Build history of the part. All positions in model axes, mm. Coordinates: 2 decimals unless noted, no trailing zeros. Loops run counter-clockwise (first coordinate to the right, second up) from the corner with the lowest first, then second, coordinate; pieces in that order, holes last.
Item 1: Drill centre lines: line 1 along Y through (x, z) = (0.75, -1); line 2 along X through (y, z) = (-4.25, -1.5); line 3 along X through (y, z) = (-6.5, -0.5). Where is each one in solid material? Low to high.
Item 2: Mould opens along Z. For faces 1 (the face through (1, 0, 4)), 2 (the face through (-0.916, -4.205, 2.908)), 3 (the face through (2.57, -4.86, -3.35)), 4 (the face through (0, -7.366, 0)) say: released by +Z, released by -Z, zero draft, split by the parting line, or undercut.
Item 3: Cut at A-A (y = -6). List the corners of the cut face in (x, z), and give its area (3 significant figures).
Item 4: Flat gauge pins, fed straight in: pin 1 (5 mm diameter, centred on x = -4, y = -7.5, fed in from +Z); pin 2 (4 mm diameter, centred on y = -1.5, z = -1, fed in from +X); pin 3 (1.9 mm diameter, centred on x = 0, z = -1, fed in from +Y); pin 4 (2 mm diameter, centred on x = -0.5, y = -5, fed in from -Z). Where does each tip first touch, or does it go through?
from build123d import *

# Parameters (mm, degrees)
FILLET1_R   = 1.524
SHELL1_T    = -1.27
SKETCH2_R   = 5.08
SKETCH2_R_2 = 3.790408203
RIM_DEPTH   = 1.524


with BuildPart() as part:
    # Sketch1 → Body (revolve)
    with BuildSketch(Plane.XY, mode=Mode.PRIVATE) as body_sk:
        Polygon((0, 0), (5.08, 0), (3.775004875, -7.400995125), (2.54, -8.636), (0, -8.636), align=None)
    revolve(body_sk.sketch.rotate(Axis((0, 0, 0), (0, -1, 0)), 90), axis=Axis((0, 0, 0), (0, -1, 0)))

    # Fillet1
    fillet1_edges = [part.edges().sort_by_distance(p)[0] for p in [
        (0, -8.636, -2.54),
        (0, -7.400995125, -3.775004875),
    ]]
    fillet(fillet1_edges, radius=FILLET1_R)

    # Shell1
    shell1_openings = [part.faces().sort_by_distance(p)[0] for p in [
        (0, 0, 0),
    ]]
    offset(amount=SHELL1_T, openings=shell1_openings, kind=Kind.INTERSECTION)

    # Sketch2 → Rim (add)
    with BuildSketch(Plane(origin=(0, 0, 0), x_dir=(-1, 0, 0), z_dir=(0, 1, 0))):
        with Locations(Location((0, 0, 0), (0, 0, 90))):
            Circle(SKETCH2_R)
        Circle(SKETCH2_R_2, mode=Mode.SUBTRACT)
    extrude(amount=-RIM_DEPTH)

    # Chamfer1: read off the stored shape, not the designer's step
    # Chamfer1 outline → Chamfer1 (revolve, cut)
    with BuildSketch(Plane.XY):
        Polygon((5.08, 0), (4.923434012, 0), (5.08, -0.181374797), align=None)
        Polygon((3.763220804, -0.154187398), (3.917408203, 0), (3.763220804, 0), align=None)
    revolve(axis=Axis((0, 0, 0), (0, 1, 0)), mode=Mode.SUBTRACT)


solid = part.part
Filled sheet:
1. line 1: y = -8.64 to -7.37
1. line 2: x = -4.06 to -2.65, 2.65 to 4.06
1. line 3: x = -3.9 to -2.6, 2.6 to 3.9
2. face 1: zero draft
2. face 2: undercut
2. face 3: split by the parting line
2. face 4: undercut
3. outline: circle Ø8.04 at (0, 0); hole circle Ø5.46 at (0, 0)
3. area: 27.4 mm2
4. pin 1: stops at z = 3.54
4. pin 2: stops at x = 5.08
4. pin 3: stops at y = -7.36
4. pin 4: stops at z = -4.36
